Check sheet for the drawn part. Datum: minimum x, y, z corner. Units: mm. Give positions to 0.01 mm unless a question says otherwise; leave off trailing zeros. Loops run counter-clockwise (first coordinate to the right, second up) from the corner with the lowest first, then second, coordinate; pieces in that order, holes last. Notation, with made-up numbers: (79.5, 51.25) - (118.5, 51.25) arc R13 ccw to (118.5, 59.25) - close; hole circle Ø5 at (45, 74.25). An arc over 180 degrees is marked (long way). Use one line per item in the form item = value.
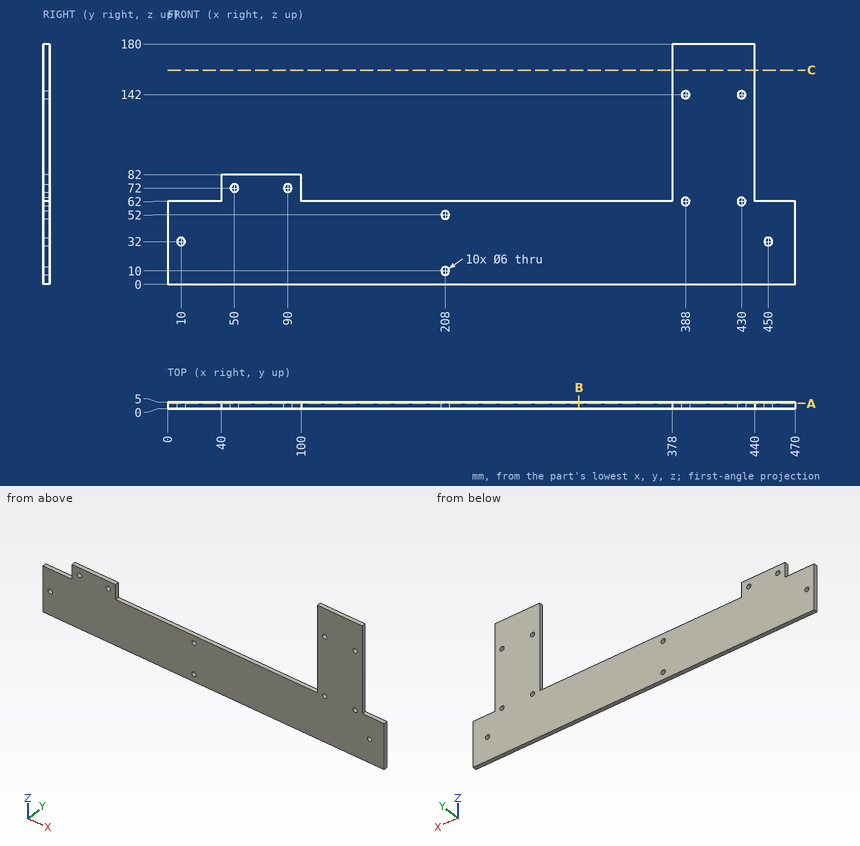
1. Section check C-C, the plane z = 160.5. Record the cut outline in (x, y).
Result set:
outline = (378, 0) - (440, 0) - (440, 5) - (378, 5) - close
2. Section check B-B, the plane x = 308. Record the cut outline in (y, z), then the cut area to 3 significant figures.
Result set:
outline = (0, 0) - (5, 0) - (5, 62) - (0, 62) - close
area = 310 mm²
3. Scan lines: probe 1 along X at (y, z) = (3.15, 142); probe 2 along Z at (x, y) = (388, 3.05); probe 3 along Z at (x, y) = (90, 3.1). Record each from-to range of solid material in increasing order.
Result set:
probe_1 = 378 to 385, 391 to 427, 433 to 440
probe_2 = 0 to 59, 65 to 139, 145 to 180
probe_3 = 0 to 69, 75 to 82
4. Section check A-A, the plane y = 4.15. State how many separate pieces and enclosed holes the cut face has, then the cut area to 3 significant figures.
Result set:
separate_pieces = 1
enclosed_holes = 10
area = 37,400 mm²
5. Depth check by flat-ended pin: pin 1 Ø2.5 at (y, z) = (3, 76) entering from -X; pin 2 Ø3 at (y, z) = (3, 90) entering from -X; pin 3 Ø2.5 at (x, y) = (78.5, 3.5) entering from +Z. Enter the tip coordinate at first touch or a pass-through.
Result set:
pin_1 = 40
pin_2 = 378
pin_3 = 82
